Autodesk Inventor part; units mm, degrees
ref_plane "YZ Plane" through (0, 0, 0) normal (1, 0, 0) x (0, 1, 0)
ref_plane "XZ Plane" through (0, 0, 0) normal (0, 1, 0) x (-1, 0, 0)
ref_plane "XY Plane" through (0, 0, 0) normal (0, 0, 1) x (1, 0, 0)
sketch "Esboço1" plane through (0, 0, 0) normal (0, 1, 0) x (-1, 0, 0)
  line L0 (-23.75, -30.48) -> (23.75, -30.48)
  line L1 (23.75, -30.48) -> (23.75, 30.48)
  line L2 (23.75, 30.48) -> (-23.75, 30.48)
  line L3 (-23.75, 30.48) -> (-23.75, -30.48)
  line L4 (-23.75, -30.48) -> (23.75, 30.48) construction
  line L5 (23.75, -30.48) -> (-23.75, 30.48) construction
  line L6 (-35, -35) -> (35, -35)
  line L7 (35, 35) -> (-35, 35)
  line L8 (-35, 35) -> (-35, -35)
  line L9 (-35, -35) -> (35, 35) construction
  line L10 (35, -35) -> (-35, 35) construction
  line L11 (23.75, 30.48) -> (20.75, 30.48)
  line L12 (23.75, 27.48) -> (23.75, 30.48)
  line L13 (-23.75, 30.48) -> (-20.75, 30.48)
  line L14 (-23.75, 27.48) -> (-23.75, 30.48)
  line L15 (-23.75, -30.48) -> (-20.75, -30.48)
  line L16 (-23.75, -27.48) -> (-23.75, -30.48)
  line L17 (23.75, -30.48) -> (20.75, -30.48)
  line L18 (23.75, -27.48) -> (23.75, -30.48)
  circle A0 centre (20.75, 27.48) radius 1.5
  circle A1 centre (-20.75, 27.48) radius 1.5
  circle A2 centre (-20.75, -27.48) radius 1.5
  circle A3 centre (20.75, -27.48) radius 1.5
  line L19 (35, -35) -> (50, -35)
  line L20 (50, -35) -> (50, 35)
  line L21 (50, 35) -> (35, 35)
  line L22 (50, -35) -> (40, -35)
  line L23 (40, -25) -> (40, 25)
  circle A4 centre (40, -25) radius 2.5
  circle A5 centre (40, 25) radius 2.5
  point P0 (0, 0)
  dimension "d0" = 47.5
  dimension "d1" = 60.96
  dimension "d12" = 3
  dimension "d13" = 3
  dimension "d33" = 15
  dimension "d34" = 70
  dimension "d35" = 10
  dimension "d36" = 10
  dimension "d37" = 50
  dimension "d38" = 5
  dimension "d39" = 5
extrude "Extrusão1" add sketch "Esboço1" along normal blind 35 contours L3 L2 L1 L0 | L8 L7 L21 L20 L19 L6 | A4 | A5
shell "Casca1" thickness 1 outward yes removed faces 5 at (6.6326, 35, -8.7485) at (19.2549, 23.3333, 27.3593) at (-22.2451, 23.3333, -27.6007) at (-22.2451, 23.3333, 27.3593) at (19.2549, 23.3333, -27.6007)
sketch "Esboço3" plane through (-50, 0, -35) normal (0, 1, 0) x (1, 0, 0)
  line L0 (0, 0) -> (85, 0)
  line L1 (0, 0) -> (10, 0)
  line L2 (10, 0) -> (10, -10)
  line L3 (10, -10) -> (10, -60)
  circle A0 centre (10, -10) radius 2.5
  circle A1 centre (10, -60) radius 2.5
  point P0 (50, -35)
  dimension "d40" = 10
  dimension "d41" = 10
  dimension "d42" = 50
  dimension "d43" = 5
  dimension "d44" = 5
extrude "Extrusão3" cut sketch "Esboço3" against normal blind 1
sketch "Esboço4" plane through (-50, 0, -35) normal (1, 0, 0) x (0, 0, -1)
  line L0 (-70, 0) -> (-70, 35)
  line L1 (-70, 35) -> (-60, 35)
  line L2 (-70, 35) -> (0, 35)
  line L3 (-60, 35) -> (-60, 25)
  line L4 (0, 0) -> (0, 35)
  line L5 (0, 35) -> (-10, 35)
  line L6 (-10, 35) -> (-10, 25)
  circle A0 centre (-60, 25) radius 2.5
  circle A1 centre (-10, 25) radius 2.5
  point P0 (-35, 0)
  dimension "d47" = 10
  dimension "d48" = 10
  dimension "d49" = 10
  dimension "d50" = 10
  dimension "d51" = 5
  dimension "d52" = 5
extrude "Extrusão4" cut sketch "Esboço4" against normal blind 1
sketch "Esboço5" plane through (0, 35, 0) normal (0, 1, 0) x (1, 0, 0)
  line L0 (-50, -35) -> (35, -35)
  line L1 (35, -35) -> (30, -35)
  line L2 (30, -35) -> (30, -30)
  line L3 (30, -30) -> (35, -30)
  line L4 (35, -30) -> (35, -35)
  line L5 (-50, -35) -> (-45, -35)
  line L6 (-45, -35) -> (-45, -30)
  line L7 (-45, -30) -> (-50, -30)
  line L8 (-50, -30) -> (-50, -35)
  circle A0 centre (-47.5, -32.5) radius 1.5
  circle A1 centre (32.5, -32.5) radius 1.5
  point P0 (0, 0)
  dimension "d63" = 5
  dimension "d64" = 5
  dimension "d65" = 5
  dimension "d66" = 5
  dimension "d67" = 3
  dimension "d68" = 3
extrude "Extrusão5" add sketch "Esboço5" against normal blind 2
thread "Rosca1"
thread "Rosca2"
thread "Rosca3"
thread "Rosca4"
sketch "Esboço9" plane through (-51, -1, 36) normal (0, 0, 1) x (1, 0, 0)
  line L0 (86, 1) -> (1, 1)
  line L1 (86, 1) -> (66, 1)
  line L2 (66, 1) -> (66, 3.5)
  circle A0 centre (66, 3.5) radius 2.5
  point P0 (51, 1)
  dimension "d101" = 20
  dimension "d102" = 2.5
extrude "Extrusão9" cut sketch "Esboço9" against normal blind 2
sketch "Esboço10" plane through (36, -1, 36) normal (1, 0, 0) x (0, 0, -1)
  line L0 (1, 34) -> (1, 36)
  line L1 (1, 36) -> (1, 21)
  line L2 (1, 1) -> (1, 34)
  line L3 (71, 1) -> (71, 36)
  circle A0 centre (26.7092, 21) radius 4.65
  line L4 (26.7092, 25.65) -> (14.7092, 25.65)
  circle A1 centre (14.7092, 21) radius 4.65
  line L5 (14.7092, 16.35) -> (26.7092, 16.35)
  circle A2 centre (58.195, 21) radius 4.65
  line L6 (58.195, 25.65) -> (46.195, 25.65)
  circle A3 centre (46.195, 21) radius 4.65
  line L7 (46.195, 16.35) -> (58.195, 16.35)
  line L8 (1, 21) -> (71, 21)
  line L9 (34.7126, 21) -> (44.7126, 21)
  point P0 (36, 1)
  dimension "d105" = 15
  dimension "d107" = 9.3
  dimension "d108" = 12
  dimension "d109" = 9.3
  dimension "d110" = 12
  dimension "d111" = 10
extrude "Extrusão10" cut sketch "Esboço10" against normal blind 2
sketch "Esboço11" plane through (-51, -1, 36) normal (0, 0, 1) x (1, 0, 0)
  circle A0 centre (66, 3.5) radius 2.5
properties part number "Caixa de Segurança_Sem fixação"
Here's how the part is built. I have some questions about the finished solid (model axes, mm). A direction names the side the tool comes from. Coordinates: 2 decimals unless noted, no trailing zeros. Write each loop counter-clockwise with the first axis right and the second up, starting at its lowest first coordinate (ties: lowest second). Pieces come first, ordered by that corner, then holes.
Item 1: I want a section at D-D on z = -2. Write out the boundary of the cut face in (x, y).
Item 2: On a 3-axis mill with a long thin cutter (end or side, diameter ignored), from which of +Z, -Z, +X, -X, +Y, -Y can I reach the whole of each face in a straight line? I mean faces 1 (the flat face through (-45, 34, 33)), 2 (the flat face through (35, 17, 0)), 3 (the cylindrical face through (-38.66, -0.49, -27.11)), 4 (the cylindrical face through (35.507, 19.898, -26.844)), 5 (the flat face through (-8, 17, 36)). Say none if no direction works.
Item 3: Will these pins go through, and if not, where does the flat tip stop? pin 1 (6 mm diameter, centred on y = 19.5, z = 16.5, fed in from +X); pin 2 (5 mm diameter, centred on x = -20.75, z = -27.48, fed in from +Y); pin 3 (4 mm diameter, centred on y = 25, z = 25, fed in from -X).
Item 4: I want a section at B-B on x = -20.75. Write out the boundary of the cut face in (y, z), and give its area (3 significant figures).
Item 5: If I drill on line 1 (Z direction, x = -50.55, y = 25); line 2 (Z direction, x = 20.75, y = -0.3); line 3 (Z direction, x = -46.5, y = 29.5), over which ranges is the centre line in solid material (lowest first)?
Item 6: I want a section at C-C on y = 20. Write out the boundary of the cut face in (x, z) (3 decimals).
Item 7: If we mould it in two halves opening along Y, with no side actions, what happens to faces 6 (the flat face through (-7, 17, -36)), 7 (the flat face through (34, 33, 31)), 8 (the cylindrical face through (35.51, 19.9, 4.64))? For each: +Y half, -Y half, draft (parallel to the pull), parting line (faces both ways), or undercut.
Item 8: I want a section at A-A on z = -13.5. Write out the boundary of the cut face in (x, y).
Findings below:
1. outline: (-51, -1) - (36, -1) - (36, 35) - (35, 35) - (35, 0) - (-50, 0) - (-50, 35) - (-51, 35) - close
2. face 1: +Y
2. face 2: none
2. face 3: +Y, -Y
2. face 4: +X
2. face 5: +Z, +X, -X, +Y, -Y
3. pin 1: stops at x = -50
3. pin 2: stops at y = 0
3. pin 3: stops at x = 35
4. outline: (-1, -36) - (35, -36) - (35, -35) - (0, -35) - (0, -28.98) - (-1, -28.98) - close; (-1, -25.98) - (0, -25.98) - (0, 25.98) - (-1, 25.98) - close; (-1, 28.98) - (0, 28.98) - (0, 35) - (35, 35) - (35, 36) - (-1, 36) - close
4. area: 136 mm2
5. line 1: z = -36 to -27.5, -22.5 to 22.5, 27.5 to 36
5. line 2: z = -36 to -28.98, -25.98 to 25.98, 28.98 to 36
5. line 3: z = -36 to -35, 35 to 36
6. outline: (-51, -36) - (36, -36) - (36, -26.845) - (35, -26.845) - (35, -35) - (-50, -35) - (-50, 35) - (35, 35) - (35, 25.941) - (36, 25.941) - (36, 36) - (-51, 36) - close; (35, -5.545) - (36, -5.545) - (36, 4.641) - (35, 4.641) - close
7. face 6: draft
7. face 7: undercut
7. face 8: undercut
8. outline: (-51, -1) - (36, -1) - (36, 15.35) - (35, 15.35) - (35, 0) - (-50, 0) - (-50, 35) - (-51, 35) - close; (35, 24.65) - (36, 24.65) - (36, 35) - (35, 35) - close
